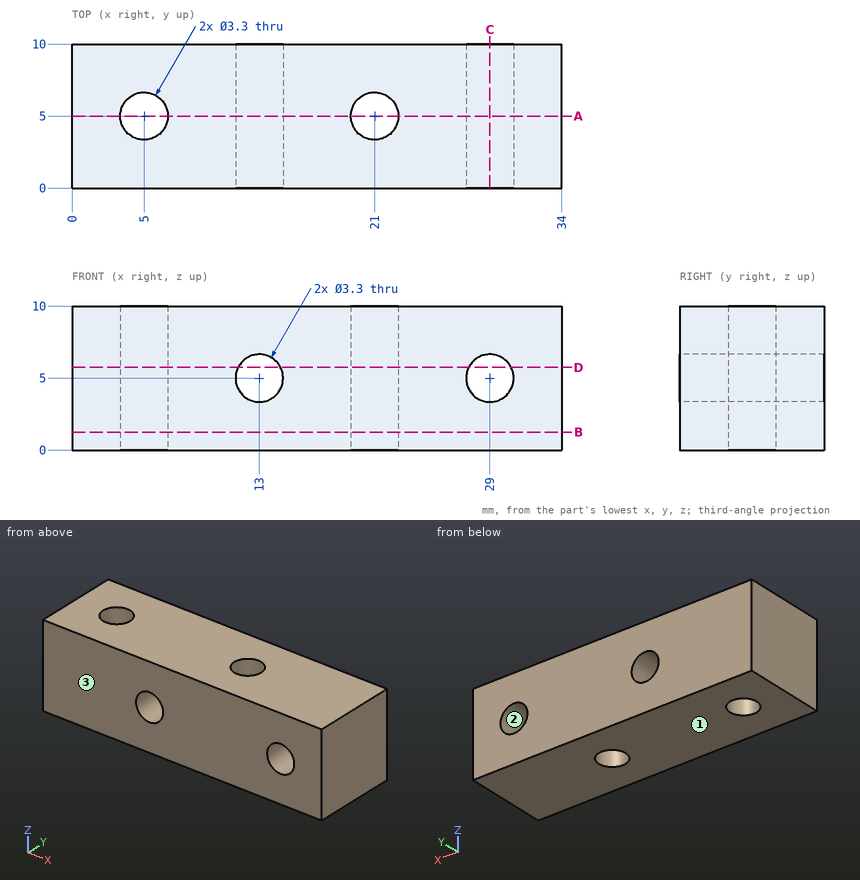
Part print with two shaded views. Sizes in mm from the minimum x, y, z corner. Round coordinates to 2 decimals unless told otherwise and drop trailing zeros. Loops run counter-clockwise (first coordinate to the right, second up) from the corner with the lowest first, then second, coordinate; pieces in that order, holes last.
1. Slice it at B-B (z = 1.25). Give the cut face in (x, y).
Solutions:
outline: (0, 0) - (34, 0) - (34, 10) - (0, 10) - close; hole circle Ø3.3 at (5, 5); hole circle Ø3.3 at (21, 5)
2. Two-plate mould, pull along Z, no slides. Class the marked faces 1, 2 and 3: pulls with the +Z half, pulls with the -Z half, needs draft (parallel to the pull), parting line crosses it, or undercut.
Solutions:
face 1: pulls with the -Z half
face 2: undercut
face 3: needs draft
3. Drill centre lines: line 1 along X through (y, z) = (6.75, 5); line 2 along Z through (x, y) = (29, 3); line 3 along X through (y, z) = (4, 0.5). Where is each one in solid material? Low to high.
Solutions:
line 1: x = 0 to 11.35, 14.65 to 27.35, 30.65 to 34
line 2: z = 0 to 3.35, 6.65 to 10
line 3: x = 0 to 3.69, 6.31 to 19.69, 22.31 to 34
4. Slice it at D-D (z = 5.75). Give the cut face in (x, y).
Solutions:
outline: (0, 0) - (11.53, 0) - (11.53, 10) - (0, 10) - close; (14.47, 0) - (27.53, 0) - (27.53, 10) - (14.47, 10) - close; (30.47, 0) - (34, 0) - (34, 10) - (30.47, 10) - close; hole circle Ø3.3 at (5, 5); hole circle Ø3.3 at (21, 5)
5. Slice it at A-A (y = 5). Give the cut face in (x, z), and give its area (3 significant figures).
Solutions:
outline: (0, 0) - (3.35, 0) - (3.35, 10) - (0, 10) - close; (6.65, 0) - (19.35, 0) - (19.35, 10) - (6.65, 10) - close; (22.65, 0) - (34, 0) - (34, 10) - (22.65, 10) - close; hole circle Ø3.3 at (13, 5); hole circle Ø3.3 at (29, 5)
area: 257 mm2
6. Slice it at C-C (x = 29). Give the cut face in (y, z), and give its area (3 significant figures).
Solutions:
outline: (0, 0) - (10, 0) - (10, 3.35) - (0, 3.35) - close; (0, 6.65) - (10, 6.65) - (10, 10) - (0, 10) - close
area: 67.0 mm2
